Design review of the part built by this model. Coordinates are the model's own, in mm. A direction names the side the tool comes from. Round coordinates to 2 decimals unless told otherwise and drop trailing zeros. Write each loop counter-clockwise with the first axis right and the second up, starting at its lowest first coordinate (ties: lowest second). Pieces come first, ordered by that corner, then holes. Notation, with made-up numbers: (58.5, -3.75) -> (70.5, -3.75) arc R38 ccw to (70.5, 35.25) -> close; hole circle Ø3 at (72.5, 41.5). An arc over 180 degrees is marked (long way). One line per question, with ' | ' between items. Start each with the question number.
1) For probe 1 along Z at (x, y) = (2.25, -5.75); probe 2 along X at (y, z) = (-2.25, -4.5) (3 decimals); probe 3 along Z at (x, y) = (-3, -4.75), list the stretches that pass through material, from the lowest coordinate up.
2) Consider section A-A (y = -5.5). Give the boundary of the cut face in (x, z) (3 decimals), then the cut area to 3 significant figures.
3) For faces 1 (the flat face through (-10.41, -3.2, -7.17)), 2 (the flat face through (-4.475, -3, -5)), 3 (the flat face through (-6, -3, 7.2)), list the 3-axis set-ups (+Z, -Z, +X, -X, +Y, -Y) from which the entire face can be reached by the end or side of a thin tool; tool diameter is ignored.
4) Consider section D-D (y = -3.25). Give the boundary of the cut face in (x, z) (3 decimals).
5) Insertion check: pin 1 Ø1.9 at (x, y) = (1.5, -1.5) entering from -Z; pin 2 Ø3 at (y, z) = (-4, -6) entering from -X; pin 3 Ø9.5 at (x, z) = (-11, -2) entering from -Y (3 decimals). Each pin has a flat end and moves straight along its axis. Give the tip position at first contact, or say it passes through.
6) Consider section B-B (z = 0.75). Give the boundary of the cut face in (x, y) (3 decimals).
7) Consider section C-C (z = 4.8). Count the separate pieces of the cut face and the enclosed holes in it, then the cut area to 3 significant figures.
8) Mouldability with a two-part tool opening along X and no side actions: class faces 4 (the flat face through (-6, -3, 6.92)), 5 (the cylindrical face through (2.39, -3.18, 6.04)), 6 (the flat face through (-10, -1.225, -8)), 7 (the flat face through (5.225, -3, 0)) as +X half, -X half, draft (parallel to the pull), parting line (faces both ways), or undercut.
```python
from build123d import *

# Parameters (mm, degrees)
F0_W      = 10.45
F0_H      = 19.9
F1_DEPTH  = 6.45
F2_W      = 6.45
F2_H      = 10
F3_DEPTH  = 0.75
F4_W      = 4
F4_H      = 0.28
F5_DEPTH  = 1
F7_DEPTH  = 4
F8_W      = 4
F8_H      = 3.6
F9_DEPTH  = 4.8
F11_D     = 2.5
F13_DEPTH = 4


with BuildPart() as f1:
    # F0 (on Front) → F1 (new body)
    with BuildSketch(Plane.XZ):
        Rectangle(F0_W, F0_H)
    extrude(amount=F1_DEPTH)

    # F2 (on face) → F3 (cut)
    with BuildSketch(Plane(origin=(-5.225, 0, 0), x_dir=(0, -1, 0), z_dir=(-1, 0, 0))):
        with Locations((3.225, -4.95)):
            Rectangle(F2_W, F2_H)
    extrude(amount=-F3_DEPTH, mode=Mode.SUBTRACT)

    # F4 (on face) → F5 (join)
    with BuildSketch(Plane(origin=(-5.225, 0, 0), x_dir=(0, -1, 0), z_dir=(-1, 0, 0))):
        with Locations((3.225, 7.06)):
            Rectangle(F4_W, F4_H)
    extrude(amount=F5_DEPTH)

    # F6 (on face) → F7 (join)
    with BuildSketch(Plane.XZ.offset(5.225)):
        with BuildLine():
            Line((-9.2832269147, -11.0147129744), (-6.225, 6.92))
            Line((-6.225, 6.92), (-6.225, 7.2))
            ThreePointArc((-6.225, 7.2), (-6.4055844086, 7.1339842783), (-6.5010158882, 6.967066224))
            Line((-6.5010158882, 6.967066224), (-9.5592428029, -10.9676467504))
            Line((-9.5592428029, -10.9676467504), (-9.2832269147, -11.0147129744))
        make_face()
    extrude(amount=-F7_DEPTH)

    # F8 (on face) → F9 (join)
    with BuildSketch(Plane(origin=(-7.4717823939, 0, 1.2740881915), x_dir=(0, -1, 0), z_dir=(-0.9857710294, 0, 0.1680936572))):
        with Locations((3.225, -10.6184365097)):
            Rectangle(F8_W, F8_H)
    extrude(amount=F9_DEPTH)

    # F11 (through all)
    with Locations(Plane.XZ.offset(6.45)):
        with Locations((2.225, -4.7), (2.225, 4.8)):
            Hole(F11_D / 2)

    # F12 (on face) → F13 (cut, through all)
    with BuildSketch(Plane.XZ.offset(5.225)):
        with BuildLine():
            Line((-13.6858065784, -6.6120214902), (-13.9883751686, -8.3864093861))
            ThreePointArc((-13.9883751686, -8.3864093861), (-13.2547207126, -7.2203479586), (-11.9114187254, -6.9145900731))
            Line((-11.9114187254, -6.9145900731), (-13.6858065784, -6.6120214902))
        make_face()
        with BuildLine():
            Line((-13.9883751686, -8.3864093861), (-14.2909437441, -10.1607971961))
            Line((-14.2909437441, -10.1607971961), (-12.5165558912, -10.463365779))
            ThreePointArc((-12.5165558912, -10.463365779), (-13.6826172757, -9.7297113304), (-13.9883751686, -8.3864093861))
        make_face()
    extrude(amount=-F13_DEPTH, mode=Mode.SUBTRACT)


solid = f1.part
```
From the geometry:
1) probe 1: z = -9.95 to -5.95, -3.45 to 3.55, 6.05 to 9.95 | probe 2: x = -8.456 to -8.172, -4.475 to 0.991, 3.459 to 5.225 | probe 3: z = -9.95 to 9.95
2) outline: (-5.225, 0.05) -> (-4.475, 0.05) -> (-4.475, -9.95) -> (5.225, -9.95) -> (5.225, 9.95) -> (-5.225, 9.95) -> close; hole circle Ø2.5 at (2.225, -4.7); hole circle Ø2.5 at (2.225, 4.8) | area: 191 mm2
3) face 1: +Z, +Y, -Y | face 2: -Z, +Y, -Y | face 3: +Z, -X, +Y, -Y
4) outline: (-12.517, -10.463) -> (-9.283, -11.015) -> (-6.225, 6.92) -> (-5.225, 6.92) -> (-5.225, 0.05) -> (-4.475, 0.05) -> (-4.475, -9.95) -> (5.225, -9.95) -> (5.225, 9.95) -> (-5.225, 9.95) -> (-5.225, 7.2) -> (-6.225, 7.2) arc R0.28 ccw to (-6.501, 6.967) -> (-8.954, -7.419) -> (-11.911, -6.915) arc R1.8 ccw to start; hole circle Ø2.5 at (2.225, -4.7); hole circle Ø2.5 at (2.225, 4.8)
5) pin 1: stops at z = -9.95 | pin 2: stops at x = -13.57 | pin 3: stops at y = -5.225
6) outline: (-7.561, -5.225) -> (-7.277, -5.225) -> (-7.277, -1.225) -> (-7.561, -1.225) -> close; (-5.225, -6.45) -> (5.225, -6.45) -> (5.225, 0) -> (-5.225, 0) -> close
7) separate pieces: 3 | enclosed holes: 0 | area: 52.4 mm2
8) face 4: undercut | face 5: undercut | face 6: draft | face 7: +X half
